The listing builds one solid part. Answer for the finished solid, in the listing's coordinates (mm). Face numbers are marked on the shaded views. A direction names the side the tool comes from. Round coordinates to 2 decimals unless told otherwise and drop trailing zeros. Write each loop counter-clockwise with the first axis right and the second up, starting at its lowest first coordinate (ties: lowest second). Pieces come first, ordered by that corner, then holes.
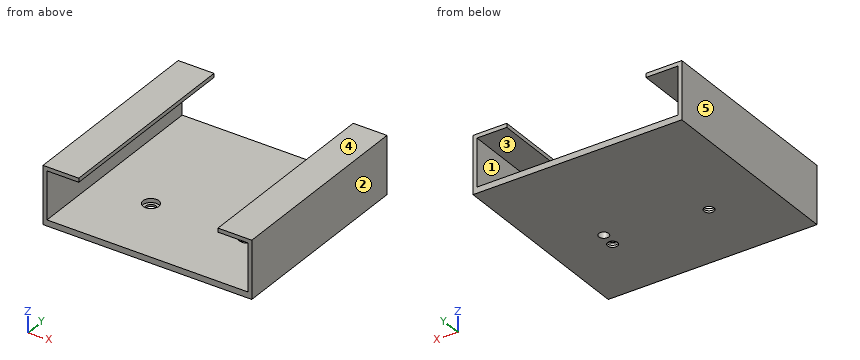
from build123d import *

# Parameters (mm, degrees)
F0_W     = 105
F0_H     = 100
F1_DEPTH = 29
F2_W     = 101
F2_H     = 24
F3_DEPTH = 110
F4_W     = 70
F4_H     = 100
F5_DEPTH = 5
F6_R     = 2.5
F7_DEPTH = 5
F8_R     = 4
F9_DEPTH = 2


with BuildPart() as f1:
    # F0 (on Top) → F1 (new body)
    with BuildSketch(Plane.XY):
        with Locations((15.428911, -27.749735)):
            Rectangle(F0_W, F0_H)
    extrude(amount=F1_DEPTH)

    # F2 (on face) → F3 (cut)
    with BuildSketch(Plane.XZ.offset(77.749735)):
        with Locations((15.428911, 15)):
            Rectangle(F2_W, F2_H)
    extrude(amount=-F3_DEPTH, mode=Mode.SUBTRACT)

    # F4 (on face) → F5 (cut)
    with BuildSketch(Plane.XY.offset(29)):
        with Locations((15.928911, -27.749735)):
            Rectangle(F4_W, F4_H)
    extrude(amount=-F5_DEPTH, mode=Mode.SUBTRACT)

    # F6 (on Top) → F7 (cut)
    with BuildSketch(Plane.XY):
        with Locations((40.928911, -34.749735)):
            Circle(F6_R)
        with Locations((41.928911, -42.749736)):
            Circle(F6_R)
        with Locations((-6.571089, -42.749736)):
            Circle(F6_R)
    extrude(amount=F7_DEPTH, mode=Mode.SUBTRACT)

    # F8 (on face) → F9 (cut)
    with BuildSketch(Plane.XY.offset(3)):
        with Locations((41.928911, -42.741511)):
            Circle(F8_R)
        with Locations((-6.599996, -42.741511)):
            Circle(F8_R)
    extrude(amount=-F9_DEPTH, mode=Mode.SUBTRACT)


solid = f1.part
1. A tool of negligible diameter and unlimited length cuts with its end or side. For the marked faces 1 and 2, from which of +Z, -Z, +X, -X, +Y, -Y can it reach the whole face along a straight path? Write none if from no direction.
Geometry says:
face 1: +Y, -Y
face 2: +Z, -Z, +X, +Y, -Y
2. Straight lines are drawn through the part: line 1 along X through (y, z) = (-16.5, 5.75); line 2 along Z through (x, y) = (52.5, -20.5); line 3 along Z through (x, y) = (4, -14.5). For each, find the intervals that lie inside material, in ascending order.
Geometry says:
line 1: x = -37.07 to -35.07, 65.93 to 67.93
line 2: z = 0 to 3, 27 to 29
line 3: z = 0 to 3
3. Section B-B on y = -19 is taken. Determine the outline of the cut face in (x, z).
Geometry says:
outline: (-37.07, 0) - (67.93, 0) - (67.93, 29) - (50.93, 29) - (50.93, 27) - (65.93, 27) - (65.93, 3) - (-35.07, 3) - (-35.07, 27) - (-19.07, 27) - (-19.07, 29) - (-37.07, 29) - close
4. Given pin 1 (4 mm diameter, centred on x = 40.93, y = -34.75, fed in from +Z); pin 2 (2.5 mm diameter, centred on x = -6.5, y = -41, fed in from +Z), each flat-ended and moving along its own axis, determine where each tip first touches the part or whether it passes through.
Geometry says:
pin 1: passes through
pin 2: stops at z = 1
5. For a pull along Z with two mould halves and no side action, classify the marked faces 3, 4 and 5 as released by +Z, released by -Z, zero draft, split by the parting line, or undercut.
Geometry says:
face 3: undercut
face 4: released by +Z
face 5: zero draft
6. Section A-A on z = 9.75 is taken. Determine the outline of the cut face in (x, y).
Geometry says:
outline: (-37.07, -77.75) - (-35.07, -77.75) - (-35.07, 22.25) - (-37.07, 22.25) - close; (65.93, -77.75) - (67.93, -77.75) - (67.93, 22.25) - (65.93, 22.25) - close
7. Section C-C on x = 4.5 is taken. Determine the outline of the cut face in (y, z).
Geometry says:
outline: (-77.75, 0) - (22.25, 0) - (22.25, 3) - (-77.75, 3) - close
